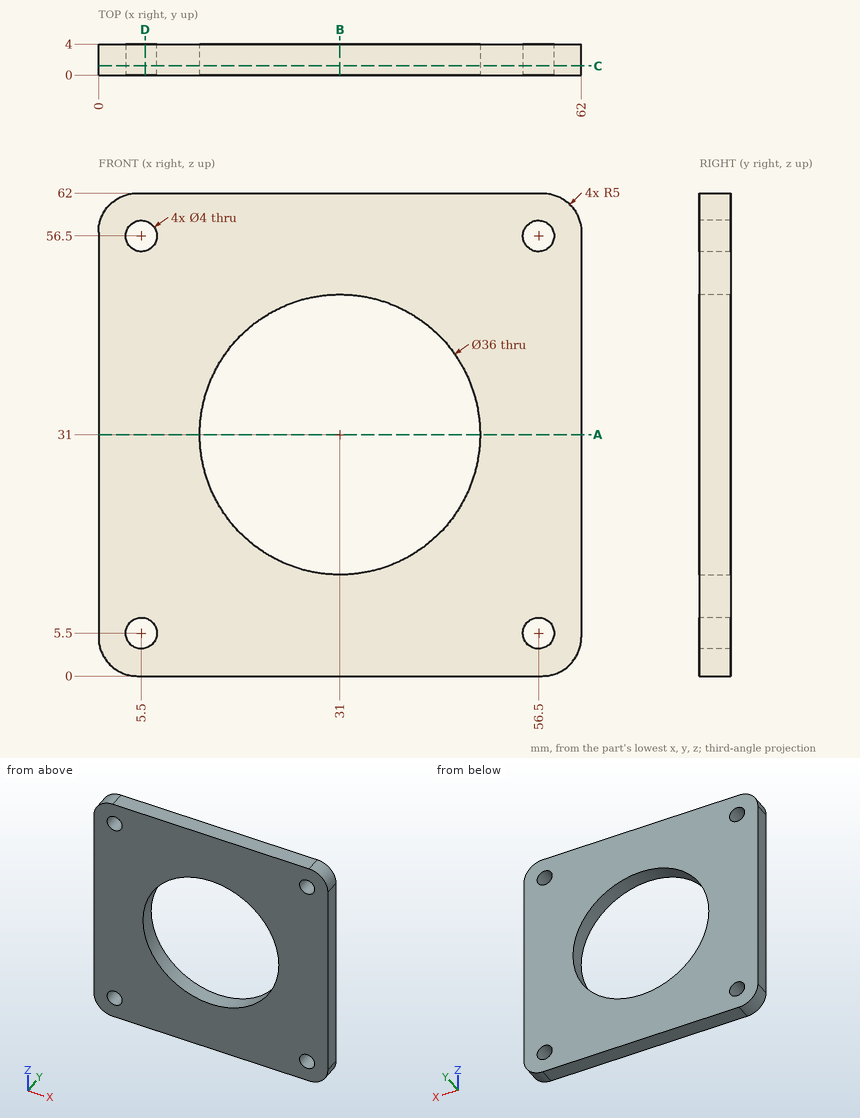
Could you check a few things on this drawing? It's one solid part, dimensions in mm from its lowest x, y, z. Coordinates: 2 decimals unless noted, no trailing zeros. Write each loop counter-clockwise with the first axis right and the second up, starting at its lowest first coordinate (ties: lowest second). Pieces come first, ordered by that corner, then holes.
1) If we section it at B-B (x = 31): List the corners of the cut face in (y, z) for me.
Filled in:
outline: (0, 0) - (4, 0) - (4, 13) - (0, 13) - close; (0, 49) - (4, 49) - (4, 62) - (0, 62) - close
2) If we section it at C-C (y = 1.2): List the corners of the cut face in (x, z) for me.
Filled in:
outline: (0, 5) arc R5 ccw to (5, 0) - (57, 0) arc R5 ccw to (62, 5) - (62, 57) arc R5 ccw to (57, 62) - (5, 62) arc R5 ccw to (0, 57) - close; hole circle Ø4 at (5.5, 5.5); hole circle Ø4 at (5.5, 56.5); hole circle Ø36 at (31, 31); hole circle Ø4 at (56.5, 5.5); hole circle Ø4 at (56.5, 56.5)
3) If we section it at D-D (x = 6): List the corners of the cut face in (y, z) for me.
Filled in:
outline: (0, 0) - (4, 0) - (4, 3.56) - (0, 3.56) - close; (0, 7.44) - (4, 7.44) - (4, 54.56) - (0, 54.56) - close; (0, 58.44) - (4, 58.44) - (4, 62) - (0, 62) - close
4) If I drill on line 1 (Z direction, x = 56.5, y = 2.35); line 2 (Z direction, x = 31, y = 2.35), over which ranges is the centre line in solid material (lowest first)?
Filled in:
line 1: z = 0 to 3.5, 7.5 to 54.5, 58.5 to 62
line 2: z = 0 to 13, 49 to 62
5) If we section it at A-A (z = 31): List the corners of the cut face in (x, y) for me, plus the area to 3 significant figures.
Filled in:
outline: (0, 0) - (13, 0) - (13, 4) - (0, 4) - close; (49, 0) - (62, 0) - (62, 4) - (49, 4) - close
area: 104 mm2
